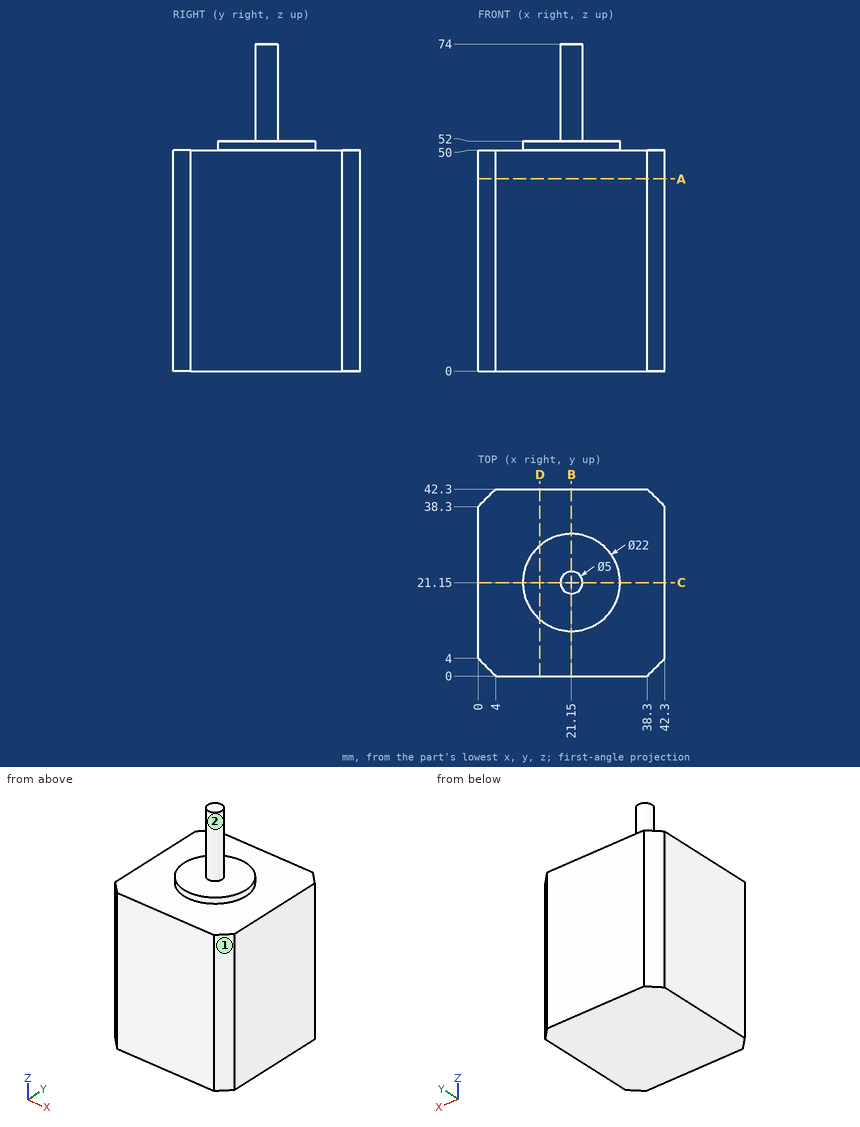
Could you check a few things on this drawing? It's one solid part, dimensions in mm from its lowest x, y, z. A direction names the side the tool comes from. Round coordinates to 2 decimals unless told otherwise and drop trailing zeros. Loops run counter-clockwise (first coordinate to the right, second up) from the corner with the lowest first, then second, coordinate; pieces in that order, holes last.
Q1. Please list where these lines run through material, in increasing order: L1, parallel to Z at x = 28, y = 10.5; L2, parallel to Z at x = 26, y = 15; L3, parallel to X at y = 39, z = 37.5.
Q2. On a 3-axis mill with a long thin cutter (end or side, diameter ignored), from which of +Z, -Z, +X, -X, +Y, -Y can I reach the whole of each face in a straight line? I mean the marked faces 1 and 2. Say none if no direction works.
Q3. I want a section at A-A (z = 43.5). Write out the boundary of the cut face in (x, y), and give its area (3 significant figures).
Q4. I want a section at B-B (x = 21.15). Write out the boundary of the cut face in (y, z), and give its area (3 significant figures).
Q5. For P1, Ø6, axis at y = 20, z = 56.5, coming from the -X side; P2, Ø2, axis at x = 14, z = 54, coming from the -Y side; P3, Ø5, axis at x = 15, y = 17, coming from the +Z side, each with a flat end and sliding along its axis, tell me the tip position at first contact or that it passes through.
Q6. I want a section at D-D (x = 14). Write out the boundary of the cut face in (y, z), and give its area (3 significant figures).
Answer below:
1. L1: z = 0 to 50
1. L2: z = 0 to 52
1. L3: x = 0.7 to 41.6
2. face 1: +Z, -Z, +X, -Y
2. face 2: +Z
3. outline: (0, 4) - (4, 0) - (38.3, 0) - (42.3, 4) - (42.3, 38.3) - (38.3, 42.3) - (4, 42.3) - (0, 38.3) - close
3. area: 1,760 mm2
4. outline: (0, 0) - (42.3, 0) - (42.3, 50) - (32.15, 50) - (32.15, 52) - (23.65, 52) - (23.65, 74) - (18.65, 74) - (18.65, 52) - (10.15, 52) - (10.15, 50) - (0, 50) - close
4. area: 2,270 mm2
5. P1: stops at x = 18.65
5. P2: passes through
5. P3: stops at z = 52
6. outline: (0, 0) - (42.3, 0) - (42.3, 50) - (29.51, 50) - (29.51, 52) - (12.79, 52) - (12.79, 50) - (0, 50) - close
6. area: 2,150 mm2
